Check sheet for the modelled part. Datum: model origin and axes. Units: mm. Face numbers are marked on the shaded views. A direction names the side the tool comes from. Round coordinates to 2 decimals unless told otherwise and drop trailing zeros. Write each loop counter-clockwise with the first axis right and the second up, starting at its lowest first coordinate (ties: lowest second). Pieces come first, ordered by that corner, then holes.
Item 1: Cross-section at A-A on x = -19. Enter the section's corners in (y, z), plus the area to 3 significant figures.
Item 2: Go/stop test with flat-tipped pins: pin 1 Ø20 at (x, z) = (37.5, 96.5) entering from +Y; pin 2 Ø20 at (x, z) = (-14, 98) entering from -Y; pin 3 Ø4 at (x, y) = (-24.5, 116) entering from +Z; pin 4 Ø10 at (x, z) = (-4.5, 153) entering from -Y. Record where each tip stops, or that it passes through.
Item 3: Cross-section at C-C on y = 109.75. Enter the section's corners in (x, z).
Item 4: Tool access check on the marked faces 1, 2, 3 and 4. Record the directions out of +Z, -Z, +X, -X, +Y, -Y that give a thin tool (end or side, any length) a straight path to the whole face; none if there is none.
Item 5: Cross-section at D-D on x = 15. Enter the section's corners in (y, z), plus the area to 3 significant figures.
Item 6: Material ranges on line 1 (X direction, y = 116.25, z = 117); line 2 (Z direction, x = -2.5, y = 116.5); line 3 (Y direction, x = -27, z = 91.5), recorded low to high.
Item 7: Cross-section at B-B on z = 105. Enter the section's corners in (x, y), plus the area to 3 significant figures.
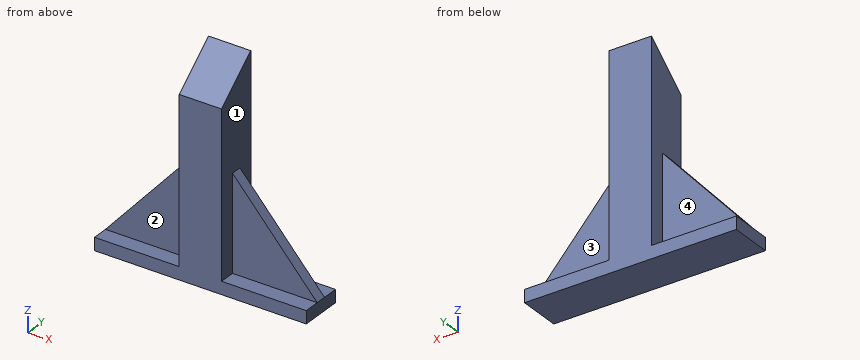
from build123d import *

# Parameters (mm, degrees)
AUFSATZ_LINEAR_AUSTRAGEN1_DEPTH = 20
SKIZZE2_W                       = 100
SKIZZE2_H                       = 6
AUFSATZ_LINEAR_AUSTRAGEN2_DEPTH = 20
AUFSATZ_LINEAR_AUSTRAGEN3_DEPTH = 2.5


with BuildPart() as part:
    # Skizze1 → Aufsatz-Linear austragen1 (new body)
    with BuildSketch(Plane.ZY):
        Polygon((75, 100), (75, 120), (175.086059804, 120), (158.405049837, 100), align=None)
    extrude(amount=-AUFSATZ_LINEAR_AUSTRAGEN1_DEPTH)

    # Skizze2 → Aufsatz-Linear austragen2 (add)
    with BuildSketch(Plane(origin=(0, 120, 0), x_dir=(1, 0, 0), z_dir=(0, 1, 0))):
        with Locations((10, -78)):
            Rectangle(SKIZZE2_W, SKIZZE2_H)
    extrude(amount=-AUFSATZ_LINEAR_AUSTRAGEN2_DEPTH)

    # Skizze3 → Aufsatz-Linear austragen3 (add, symmetric)
    with BuildSketch(Plane(origin=(0, 110, 0), x_dir=(1, 0, 0), z_dir=(0, 1, 0))):
        Polygon((-40, -81), (0, -126.018077963), (20, -126.018077963), (60, -81), align=None)
    extrude(amount=AUFSATZ_LINEAR_AUSTRAGEN3_DEPTH, both=True)


solid = part.part
Response values:
1. outline: (100, 75) - (120, 75) - (120, 81) - (112.5, 81) - (112.5, 104.63) - (107.5, 104.63) - (107.5, 81) - (100, 81) - close
1. area: 238 mm2
2. pin 1: stops at y = 112.5
2. pin 2: stops at y = 107.5
2. pin 3: stops at z = 81
2. pin 4: stops at y = 100
3. outline: (-40, 75) - (60, 75) - (60, 81) - (20, 126.02) - (20, 166.54) - (0, 166.54) - (0, 126.02) - (-40, 81) - close
4. face 1: +Z, +X
4. face 2: +Z, -X, -Y
4. face 3: +Z, +X, +Y
4. face 4: +Z, -X, +Y
5. outline: (100, 75) - (120, 75) - (120, 175.09) - (100, 158.41) - close
5. area: 1,830 mm2
6. line 1: x = 0 to 20
6. line 2: z = 75 to 81
6. line 3: y = 107.5 to 112.5
7. outline: (-18.68, 107.5) - (0, 107.5) - (0, 100) - (20, 100) - (20, 107.5) - (38.68, 107.5) - (38.68, 112.5) - (20, 112.5) - (20, 120) - (0, 120) - (0, 112.5) - (-18.68, 112.5) - close
7. area: 587 mm2
